Autodesk Inventor part; units mm, degrees
ref_plane "YZ Plane" through (0, 0, 0) normal (1, 0, 0) x (0, 1, 0)
ref_plane "XZ Plane" through (0, 0, 0) normal (0, 1, 0) x (-1, 0, 0)
ref_plane "XY Plane" through (0, 0, 0) normal (0, 0, 1) x (1, 0, 0)
sketch "Sketch1" plane through (0, 0, 0) normal (0, 1, 0) x (-1, 0, 0)
  circle A0 centre (0, 0) radius 7.747
  dimension "d0" = 15.494
extrude "Extrusion1" add sketch "Sketch1" along normal blind 21.0058
sketch "Sketch2" plane through (0, 0, 0) normal (1, 0, 0) x (0, 1, 0)
  line L0 (5.08, 0) -> (7.62, 0)
  line L1 (7.62, 0) -> (7.62, -10.3124)
  line L2 (7.62, -10.3124) -> (5.08, -10.3124)
  line L3 (5.08, -10.3124) -> (5.08, 0)
  line L4 (0, 7.747) -> (0, -7.747)
  point P0 (0, 0)
  dimension "d3" = 10.3124
  dimension "d4" = 5.08
  dimension "d5" = 2.54
revolve "Revolution1" add sketch "Sketch2" angle 360 about axis through (0, 5.08, 0) along (0, 1, 0)
sketch "Sketch3" plane through (0, 0, 0) normal (0, -1, 0) x (1, 0, 0)
  circle A0 centre (0, 0) radius 7.747
  circle A1 centre (0, 0) radius 4.8747
extrude "Extrusion2" add sketch "Sketch3" along normal blind 5.588 contours A1
sketch "Sketch4" plane through (0, 21.0058, 0) normal (0, 1, 0) x (1, 0, 0)
  circle A0 centre (0, 0) radius 7.747
  circle A1 centre (0, 0) radius 6.35
  dimension "d9" = 12.7
extrude "Extrusion3" cut sketch "Sketch4" against normal blind 5.588 contours A1
properties part number "BiglConnector"
Geometry check sheet. Reference: the model listing, model coordinates, mm. A direction names the side the tool comes from. Coordinates: 2 decimals unless noted, no trailing zeros. Order: outer loops, then holes, each group sorted by start corner. A loop starts at its lowest first (then second) coordinate and runs counter-clockwise, first axis right, second up. Notation, with made-up numbers: (11, -11) - (53, -11) arc R17 cw to (53, 17) - close; hole circle Ø6 at (30, 11.5). An arc over 180 degrees is marked (long way). One line per item, written item: value.
(1) Thickness scan on probe 1 along X at (y, z) = (18.85, 0); probe 2 along Y at (x, z) = (1.5, 5.75). Record the ranges inside material, lowest first. Write a range as from..to.
Data:
probe 1: x = -7.75..-6.35, 6.35..7.75
probe 2: y = 0..15.42
(2) Sectioned sample at C-C (y = 12.5). Enter the section's corners in (x, z).
Data:
outline: circle Ø15.49 at (0, 0)
(3) Depth check by flat-ended pin: pin 1 Ø12 at (x, z) = (-7.5, -3.5) entering from +Y; pin 2 Ø1 at (x, y) = (-5, 4) entering from -Z; pin 3 Ø4 at (x, z) = (3.5, 7.5) entering from -Y; pin 4 Ø1 at (y, z) = (11, -7) entering from -X (3 decimals). Enter the tip coordinate at first touch or a pass-through.
Data:
pin 1: stops at y = 21.01
pin 2: stops at z = -6.31
pin 3: stops at y = 0
pin 4: stops at x = -4.215
(4) Sectioned sample at D-D (z = 6). Enter the section's corners in (x, y), and give its area (3 significant figures).
Data:
outline: (-8.39, 5.08) - (-4.9, 5.08) - (-4.9, 0) - (4.9, 0) - (4.9, 5.08) - (8.39, 5.08) - (8.39, 7.62) - (4.9, 7.62) - (4.9, 21.01) - (2.08, 21.01) - (2.08, 15.42) - (-2.08, 15.42) - (-2.08, 21.01) - (-4.9, 21.01) - (-4.9, 7.62) - (-8.39, 7.62) - close
area: 200 mm^2
(5) Sectioned sample at A-A (x = 0). Enter the section's corners in (y, z), and give its area (3 significant figures).
Data:
outline: (-5.59, -4.87) - (0, -4.87) - (0, -7.75) - (5.08, -7.75) - (5.08, -10.31) - (7.62, -10.31) - (7.62, -7.75) - (21.01, -7.75) - (21.01, -6.35) - (15.42, -6.35) - (15.42, 6.35) - (21.01, 6.35) - (21.01, 7.75) - (7.62, 7.75) - (7.62, 10.31) - (5.08, 10.31) - (5.08, 7.75) - (0, 7.75) - (0, 4.87) - (-5.59, 4.87) - close
area: 322 mm^2
(6) Release check for a two-part mould opening along Z. For faces 1 (the face through (-4.165, 14.219, -6.532)), 2 (the face through (-8, 7.62, -1)), 3 (the face through (-1.38, 18.25, 6.2)) record: +Z half, -Z half, draft (parallel to the pull), parting line (faces both ways), or undercut.
Data:
face 1: parting line
face 2: draft
face 3: undercut
(7) Sectioned sample at B-B (z = 0). Enter the section's corners in (x, y), and give its area (3 significant figures).
Data:
outline: (-10.31, 5.08) - (-7.75, 5.08) - (-7.75, 0) - (-4.87, 0) - (-4.87, -5.59) - (4.87, -5.59) - (4.87, 0) - (7.75, 0) - (7.75, 5.08) - (10.31, 5.08) - (10.31, 7.62) - (7.75, 7.62) - (7.75, 21.01) - (6.35, 21.01) - (6.35, 15.42) - (-6.35, 15.42) - (-6.35, 21.01) - (-7.75, 21.01) - (-7.75, 7.62) - (-10.31, 7.62) - close
area: 322 mm^2
(8) Access from +Z, -Z, +X, -X, +Y, -Y to the whole of each face (thin tool, end or side, straight path). Record for faces 4 (the face through (6, 21.006, 3)), 5 (the face through (-8, 5.08, -1)), 6 (the face through (0, 15.418, 0)).
Data:
face 4: +Z, -Z, +X, -X, +Y
face 5: -Y
face 6: +Y
